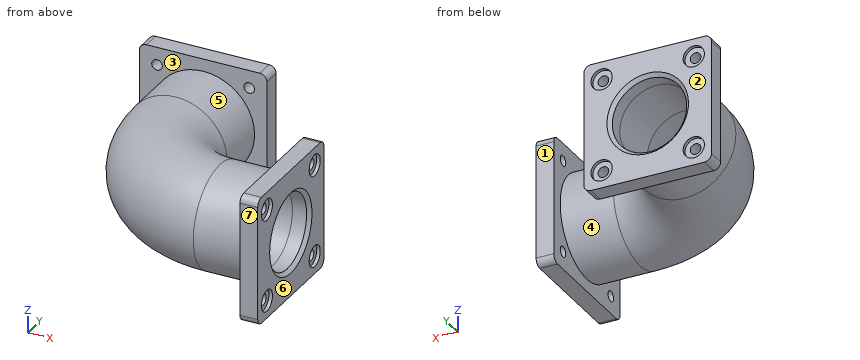
from build123d import *
from build123d.topology import SkipClean

# Parameters (mm, degrees)
SKETCH3_W           = 360
SKETCH3_H           = 360
SKETCH3_R           = 30
SKETCH3_R_2         = 145
SKETCH3_R_3         = 105
BOSS_EXTRUDE1_DEPTH = 50
SKETCH3_3_R         = 30
SKETCH3_3_R_2       = 15
BOSS_EXTRUDE2_DEPTH = 40
SKETCH2_W           = 360
SKETCH2_H           = 360
SKETCH2_R           = 30
SKETCH2_R_2         = 145
SKETCH2_R_3         = 105
BOSS_EXTRUDE3_DEPTH = 50
SKETCH2_3_R         = 30
SKETCH2_3_R_2       = 15
BOSS_EXTRUDE4_DEPTH = 40
SKETCH4_R           = 145
SKETCH5_R           = 105
CHAMFER1_SIZE       = 10
FILLET1_R           = 20
FILLET2_R           = 20


with BuildPart() as part:
    # Sketch3 → Boss-Extrude1 (new body)
    # profile 1 of 2: a face of its own
    with BuildSketch(Plane(origin=(410, 0, 0), x_dir=(0, 0, -1), z_dir=(1, 0, 0))):
        Rectangle(SKETCH3_W, SKETCH3_H)
        with Locations((-130, 130)):
            Circle(SKETCH3_R, mode=Mode.SUBTRACT)
        with Locations((-130, -130)):
            Circle(SKETCH3_R, mode=Mode.SUBTRACT)
        with Locations((130, -130)):
            Circle(SKETCH3_R, mode=Mode.SUBTRACT)
        with Locations((130, 130)):
            Circle(SKETCH3_R, mode=Mode.SUBTRACT)
        Circle(SKETCH3_R_2, mode=Mode.SUBTRACT)
    # profile 2 of 2: a face of its own
    with BuildSketch(Plane(origin=(410, 0, 0), x_dir=(0, 0, -1), z_dir=(1, 0, 0))):
        Circle(SKETCH3_R_2)
        Circle(SKETCH3_R_3, mode=Mode.SUBTRACT)
    extrude(amount=BOSS_EXTRUDE1_DEPTH)

    # Sketch3_3 → Boss-Extrude2 (add)
    # profile 1 of 4: a face of its own
    with BuildSketch(Plane(origin=(410, 0, 0), x_dir=(0, 0, -1), z_dir=(1, 0, 0))):
        with Locations((-130, 130)):
            Circle(SKETCH3_3_R)
        with Locations((-130, 130)):
            Circle(SKETCH3_3_R_2, mode=Mode.SUBTRACT)
    # profile 2 of 4: a face of its own
    with BuildSketch(Plane(origin=(410, 0, 0), x_dir=(0, 0, -1), z_dir=(1, 0, 0))):
        with Locations((130, 130)):
            Circle(SKETCH3_3_R)
        with Locations((130, 130)):
            Circle(SKETCH3_3_R_2, mode=Mode.SUBTRACT)
    # profile 3 of 4: a face of its own
    with BuildSketch(Plane(origin=(410, 0, 0), x_dir=(0, 0, -1), z_dir=(1, 0, 0))):
        with Locations((-130, -130)):
            Circle(SKETCH3_3_R)
        with Locations((-130, -130)):
            Circle(SKETCH3_3_R_2, mode=Mode.SUBTRACT)
    # profile 4 of 4: a face of its own
    with BuildSketch(Plane(origin=(410, 0, 0), x_dir=(0, 0, -1), z_dir=(1, 0, 0))):
        with Locations((130, -130)):
            Circle(SKETCH3_3_R)
        with Locations((130, -130)):
            Circle(SKETCH3_3_R_2, mode=Mode.SUBTRACT)
    extrude(amount=BOSS_EXTRUDE2_DEPTH)



with BuildPart() as body_2:
    # Sketch2 → Boss-Extrude3 (new body)
    # profile 1 of 2: a face of its own
    with BuildSketch(Plane(origin=(0, 410, 0), x_dir=(1, 0, 0), z_dir=(0, 1, 0))):
        Rectangle(SKETCH2_W, SKETCH2_H)
        with Locations(Location((-130, 130, 0), (0, 0, 270))):
            Circle(SKETCH2_R, mode=Mode.SUBTRACT)
        with Locations(Location((-130, -130, 0), (0, 0, 270))):
            Circle(SKETCH2_R, mode=Mode.SUBTRACT)
        with Locations(Location((130, -130, 0), (0, 0, 270))):
            Circle(SKETCH2_R, mode=Mode.SUBTRACT)
        with Locations(Location((130, 130, 0), (0, 0, 270))):
            Circle(SKETCH2_R, mode=Mode.SUBTRACT)
        Circle(SKETCH2_R_2, mode=Mode.SUBTRACT)
    # profile 2 of 2: a face of its own
    with BuildSketch(Plane(origin=(0, 410, 0), x_dir=(1, 0, 0), z_dir=(0, 1, 0))):
        Circle(SKETCH2_R_2)
        with Locations(Location((0, 0, 0), (0, 0, 270))):
            Circle(SKETCH2_R_3, mode=Mode.SUBTRACT)
    extrude(amount=BOSS_EXTRUDE3_DEPTH)

    # Sketch2_3 → Boss-Extrude4 (add)
    # profile 1 of 4: a face of its own
    with BuildSketch(Plane(origin=(0, 410, 0), x_dir=(1, 0, 0), z_dir=(0, 1, 0))):
        with Locations(Location((-130, -130, 0), (0, 0, 270))):
            Circle(SKETCH2_3_R)
        with Locations(Location((-130, -130, 0), (0, 0, 270))):
            Circle(SKETCH2_3_R_2, mode=Mode.SUBTRACT)
    # profile 2 of 4: a face of its own
    with BuildSketch(Plane(origin=(0, 410, 0), x_dir=(1, 0, 0), z_dir=(0, 1, 0))):
        with Locations(Location((-130, 130, 0), (0, 0, 270))):
            Circle(SKETCH2_3_R)
        with Locations(Location((-130, 130, 0), (0, 0, 270))):
            Circle(SKETCH2_3_R_2, mode=Mode.SUBTRACT)
    # profile 3 of 4: a face of its own
    with BuildSketch(Plane(origin=(0, 410, 0), x_dir=(1, 0, 0), z_dir=(0, 1, 0))):
        with Locations(Location((130, -130, 0), (0, 0, 270))):
            Circle(SKETCH2_3_R)
        with Locations(Location((130, -130, 0), (0, 0, 270))):
            Circle(SKETCH2_3_R_2, mode=Mode.SUBTRACT)
    # profile 4 of 4: a face of its own
    with BuildSketch(Plane(origin=(0, 410, 0), x_dir=(1, 0, 0), z_dir=(0, 1, 0))):
        with Locations(Location((130, 130, 0), (0, 0, 270))):
            Circle(SKETCH2_3_R)
        with Locations(Location((130, 130, 0), (0, 0, 270))):
            Circle(SKETCH2_3_R_2, mode=Mode.SUBTRACT)
    extrude(amount=BOSS_EXTRUDE4_DEPTH)


with BuildPart() as part_1:
    add(part.part)

    add(body_2.part)  # Sweep1 merges body 2
    # Sweep1: sweep along a path in Sketch1
    with BuildLine(Plane.XY) as sweep1_path:
        Line((0, 410), (0, 260))
        ThreePointArc((0, 260), (76.152236891, 76.152236891), (260, 0))
        Line((260, 0), (410, 0))
    # Sketch4 → Sweep1 (sweep)
    with BuildSketch(Plane.ZY.offset(-410)):
        Circle(SKETCH4_R)
    sweep(path=sweep1_path.line)

    # Cut-Sweep2: sweep along a path in Sketch6
    with SkipClean():  # the faces are left unmerged after this step: merging them gives an invalid solid
        with BuildLine(Plane.XY) as cut_sweep2_path:
            Line((0, 410), (0, 260))
            ThreePointArc((0, 260), (76.152236891, 76.152236891), (260, 0))
            Line((260, 0), (410, 0))
        # Sketch5 → Cut-Sweep2 (sweep, cut)
        with BuildSketch(Plane(origin=(0, 410, 0), x_dir=(1, 0, 0), z_dir=(0, 1, 0))):
            Circle(SKETCH5_R)
        sweep(path=cut_sweep2_path.line, mode=Mode.SUBTRACT)

    # Chamfer1
    chamfer1_edges = [part_1.edges().sort_by_distance(p)[0] for p in [
        (460, 0, 105),
        (0, 460, -105),
    ]]
    chamfer(chamfer1_edges, length=CHAMFER1_SIZE)

    # Fillet1
    fillet1_edges = [part_1.edges().sort_by_distance(p)[0] for p in [
        (-180, 435, 180),
    ]]
    fillet(fillet1_edges, radius=FILLET1_R)

    # Fillet2
    fillet2_edges = [part_1.edges().sort_by_distance(p)[0] for p in [
        (435, -180, -180),
        (435, -180, 180),
        (435, 180, 180),
        (435, 180, -180),
        (180, 435, 180),
        (180, 435, -180),
        (-180, 435, -180),
    ]]
    fillet(fillet2_edges, radius=FILLET2_R)


solid = part_1.part
The model under review builds one solid part; all positions refer to its coordinate system, in mm. Face numbers are marked on the shaded views. A direction names the side the tool comes from. Round coordinates to 2 decimals unless told otherwise and drop trailing zeros. Order: outer loops, then holes, each group sorted by start corner. A loop starts at its lowest first (then second) coordinate and runs counter-clockwise, first axis right, second up. Notation, with made-up numbers: (41.25, -1.75) - (68.25, -1.75) arc R16 ccw to (68.25, 3.25) - close; hole circle Ø2 at (19, -6). An arc over 180 degrees is marked (long way). Use one line per item in the form item = value.
Q1. To check wall thickness, follow line 1 (Y direction, x = 426, z = 130); line 2 (Y direction, x = 455.5, z = 130). State the ranges of each line that lie inside material, in increasing order.
Response values:
line_1 = -180 to -145, -115 to 115, 145 to 180
line_2 = -180 to -160, -100 to 100, 160 to 180
Q2. Mouldability with a two-part tool opening along Y and no side actions: class the marked faces 4, 5, 6 and 7 as pulls with the +Y half, pulls with the -Y half, needs draft (parallel to the pull), parting line crosses it, or undercut.
Response values:
face_4 = parting line crosses it
face_5 = undercut
face_6 = needs draft
face_7 = pulls with the -Y half
Q3. Add section B-B on y = 360.5. Give the boundary of the cut face in (x, z), then the cut area to 3 significant figures.
Response values:
outline = circle Ø290 at (0, 0); hole circle Ø210 at (0, 0)
area = 31,400 mm^2
Q4. Add section D-D on y = 130. Give the number of separate pieces and of enclosed holes in the cut face, then the cut area to 3 significant figures.
Response values:
separate_pieces = 3
enclosed_holes = 1
area = 78,000 mm^2
Q5. Add section A-A on z = 0. Give the boundary of the cut face in (x, y), then the cut area to 3 significant figures.
Response values:
outline = (-180, 410) - (-145, 410) - (-145, 260) arc R405 ccw to (260, -145) - (410, -145) - (410, -180) - (460, -180) - (460, -115) - (450, -105) - (260, -105) arc R365 cw to (-105, 260) - (-105, 450) - (-115, 460) - (-180, 460) - close; (105, 260) arc R155 ccw to (260, 105) - (450, 105) - (460, 115) - (460, 180) - (410, 180) - (410, 145) - (260, 145) arc R115 cw to (145, 260) - (145, 410) - (180, 410) - (180, 460) - (115, 460) - (105, 450) - close
area = 71,500 mm^2
Q6. Tool access review of the marked faces 1, 2 and 3: name each direction out of +Z, -Z, +X, -X, +Y, -Y from which nothing blocks a thin tool from reaching the whole face with its end or side.
Response values:
face_1 = +Z, -Z, +X, +Y
face_2 = +Z, -Z, +X, -X, +Y
face_3 = none
Q7. Clearance check with flat-ended pins moving along their axes: P1, Ø1, axis at x = 263, z = 58.5, coming from the +Y side; P2, Ø4, axis at x = -47.5, y = 395, coming from the +Z side; P3, Ø6, axis at x = 116.5, z = 136.5, coming from the +Y side. State where each tip first meets the part, or that it passes through.
Response values:
P1 = 132.89
P2 = 137.68
P3 = 450
